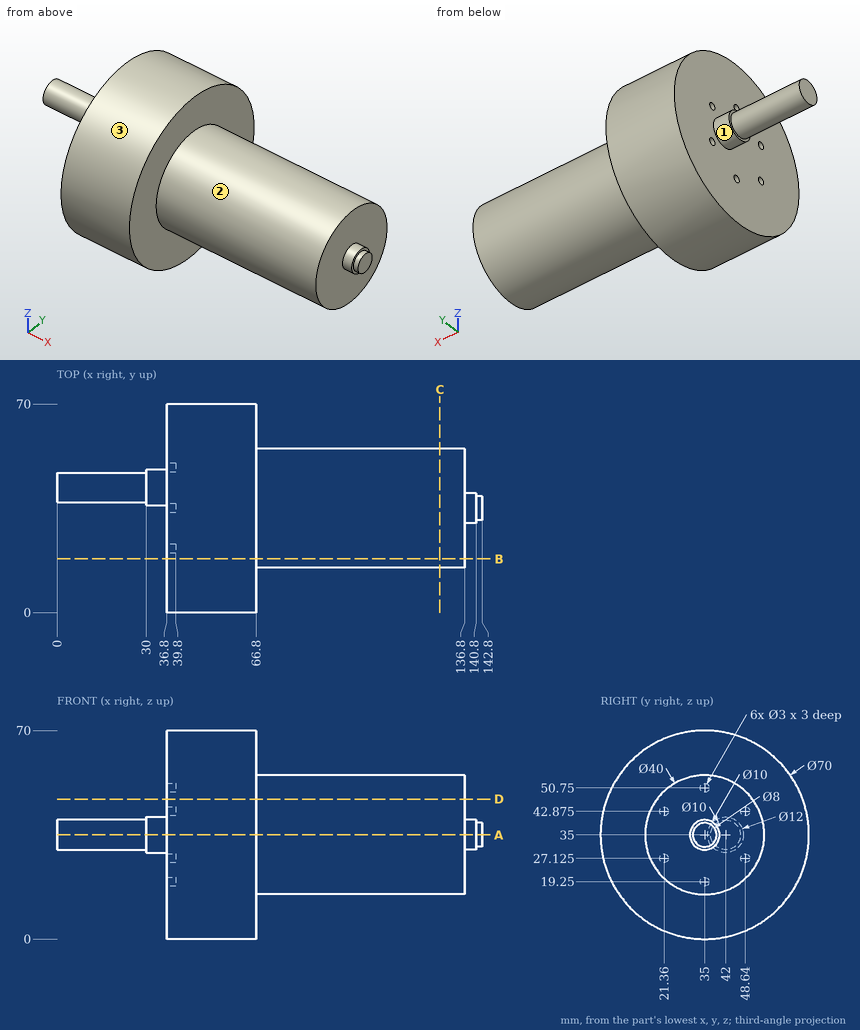
Study the drawing (mm; zero at the part's minimum x, y, z) and answer. A direction names the side the tool comes from. Give positions to 0.01 mm unless a question says otherwise; leave off trailing zeros. Write each loop counter-clockwise with the first axis right and the second up, starting at its lowest first coordinate (ties: lowest second). Pieces come first, ordered by that corner, then holes.
Item 1: Section A-A, the plane z = 35 is taken. Write down the section's boundary in (x, y).
Item 2: Which of the six approach directions +Z, -Z, +X, -X, +Y, -Y give full straight-line access (tool end or side, diameter ignored) to the marked faces 1, 2 and 3?
Item 3: Flat-ended cylindrical pins translate along their axes: P1, Ø10, axis at x = 46.5, y = 36, coming from the +Z side; P2, Ø0.9, axis at y = 49, z = 42.5, coming from the -X side; P3, Ø5, axis at y = 25.5, z = 48.5, coming from the +X side. Find the tip coordinate at first contact, or state that the pin passes through.
Item 4: Section B-B, the plane y = 18 is taken. Write down the section's boundary in (x, z).
Item 5: Find the intervals of material crossed by line 1 along X through (y, z) = (51.5, 7); line 2 along Z through (x, y) = (41, 34); line 3 along X through (y, z) = (24, 51), in increasing order.
Item 6: Section D-D, the plane z = 47 is taken. Write down the section's boundary in (x, y), plus the area to 3 significant figures.
Item 7: Section C-C, the plane x = 128.5 is taken. Write down the section's boundary in (y, z).
Completed:
1. outline: (0, 37) - (30, 37) - (30, 36) - (36.8, 36) - (36.8, 0) - (66.8, 0) - (66.8, 15) - (136.8, 15) - (136.8, 30) - (140.8, 30) - (140.8, 31) - (142.8, 31) - (142.8, 39) - (140.8, 39) - (140.8, 40) - (136.8, 40) - (136.8, 55) - (66.8, 55) - (66.8, 70) - (36.8, 70) - (36.8, 48) - (30, 48) - (30, 47) - (0, 47) - close
2. face 1: -X
2. face 2: +X
2. face 3: +X, -X
3. P1: stops at z = 70
3. P2: stops at x = 39.8
3. P3: stops at x = 136.8
4. outline: (36.8, 4.41) - (66.8, 4.41) - (66.8, 24.46) - (136.8, 24.46) - (136.8, 45.54) - (66.8, 45.54) - (66.8, 65.59) - (36.8, 65.59) - close
5. line 1: x = 36.8 to 66.8
5. line 2: z = 0.01 to 69.99
5. line 3: x = 36.8 to 136.8
6. outline: (36.8, 2.12) - (66.8, 2.12) - (66.8, 19) - (136.8, 19) - (136.8, 51) - (66.8, 51) - (66.8, 67.88) - (36.8, 67.88) - close
6. area: 4,210 mm2
7. outline: circle Ø40 at (35, 35)
